from build123d import *

# Parameters (mm, degrees)
BOSS_EXTRUDE2_DEPTH = 32
CUT_EXTRUDE2_DEPTH  = 2
CHAMFER3_SIZE       = 2
CUT_EXTRUDE3_DEPTH  = 2
BOSS_EXTRUDE4_DEPTH = 2
CHAMFER4_SIZE       = 2
CUT_EXTRUDE4_DEPTH  = 2
CUT_EXTRUDE5_DEPTH  = 30


with BuildPart() as part:
    # Sketch1 → Boss-Extrude2 (new body)
    with BuildSketch(Plane(origin=(0, 0, 0), x_dir=(1, 0, 0), z_dir=(0, 1, 0))):
        Polygon((-46.372280014218745, 14.680854952562456), (-42.04215299529653, 12.180854952562488), (-43.04215299529651, 10.448804144993609), (-47.372280014218724, 12.948804144993577), (-48.37228001421871, 11.216753337424702), (-36.60670775986293, 4.423897029202528), (1.0929e-13, -2.030853223771254), (36.60670775986312, 4.423897029202558), (48.37228001421891, 11.216753337424812), (47.37228001421898, 12.948804144993561), (43.04215299529678, 10.448804144993572), (42.04215299529679, 12.180854952562449), (46.37228001421899, 14.680854952562438), (45.372280014219, 16.412905760131313), (40, 13.31121844775995), (40, 8.692416294243028), (35.91211504919529, 6.332274817479665), (0, 0), (-35.91211504919526, 6.3322748174796235), (-40.00000000000001, 8.692416294243028), (-40.00000000000001, 13.311218447759854), (-45.37228001421887, 16.41290576013115), align=None)
    extrude(amount=BOSS_EXTRUDE2_DEPTH)

    # Sketch9 → Cut-Extrude2 (cut)
    with BuildSketch(Plane(origin=(6.236073334457828, 0, 10.801195855006485), x_dir=(-0.8660254037844402, 0, 0.4999999999999974), z_dir=(-0.4999999999999974, 0, -0.8660254037844402))):
        Polygon((-44.8209624184392, 20), (-47.50000000000022, 7.944330883818674), (-47.50000000000013, 32), (-44.8209624184392, 32), align=None)
    extrude(amount=-CUT_EXTRUDE2_DEPTH, mode=Mode.SUBTRACT)

    # Chamfer3
    chamfer3_edges = [part.edges().sort_by_distance(p)[0] for p in [
        (47.872280014218944, 0, -12.082778741209186),
        (-47.87228001421872, 0, -12.08277874120914),
    ]]
    chamfer(chamfer3_edges, length=CHAMFER3_SIZE)

    # Sketch8 → Cut-Extrude3 (cut)
    with BuildSketch(Plane(origin=(-6.236073334457578, 0, 10.801195855006183), x_dir=(-0.8660254037844388, 0, -0.49999999999999983), z_dir=(0.4999999999999998, 0, -0.8660254037844387))):
        Polygon((44.82096241843918, 32), (47.50000000000006, 32), (47.50000000000006, 7.944330883819361), (44.82096241843918, 20), align=None)
    extrude(amount=-CUT_EXTRUDE3_DEPTH, mode=Mode.SUBTRACT)

    # Sketch11 → Boss-Extrude4 (add)
    with BuildSketch(Plane(origin=(0, 32, 0), x_dir=(1, 0, 0), z_dir=(0, 1, 0))):
        Polygon((-46.37228001421867, 14.680854952562523), (-45.37228001421879, 16.4129057601312), (-40.00000000000001, 13.311218447759854), (-1.3184e-13, 6.258139219421286), (40, 13.31121844775995), (45.37228001421892, 16.412905760131267), (46.372280014218916, 14.680854952562392), (45.052165410893835, 11.609285354213014), (46.05216541089376, 9.87723454664427), (36.60670775986312, 4.423897029202558), (1.0929e-13, -2.030853223771254), (-36.60670775986293, 4.423897029202528), (-46.052165410893714, 9.877234546644353), (-45.0521654108937, 11.609285354213252), align=None)
    extrude(amount=BOSS_EXTRUDE4_DEPTH)

    # Chamfer4
    chamfer4_edges = [part.edges().sort_by_distance(p)[0] for p in [
        (18.303353879931613, 34, -1.1965219027156522),
        (-18.303353879931407, 34, -1.1965219027156366),
        (41.32943658537844, 34, -7.150565787923414),
        (-41.32943658537832, 34, -7.1505657879234406),
    ]]
    chamfer(chamfer4_edges, length=CHAMFER4_SIZE)

    # Sketch12 → Cut-Extrude4 (cut)
    with BuildSketch(Plane.XZ):
        Polygon((40, -8.692416294243028), (43.04215299529678, -10.448804144993572), (47.37228001421891, -12.948804144993517), (45.37228001421892, -16.412905760131267), (40, -13.31121844775995), align=None)
        Polygon((-47.37228001421867, -12.948804144993655), (-40.00000000000001, -8.692416294243028), (-40.00000000000001, -13.311218447759854), (-45.37228001421879, -16.4129057601312), align=None)
    extrude(amount=-CUT_EXTRUDE4_DEPTH, mode=Mode.SUBTRACT)

    # Sketch13 → Cut-Extrude5 (cut)
    with BuildSketch(Plane.XZ.offset(-2)):
        Polygon((43.04215299529678, -10.448804144993572), (42.04215299529679, -12.180854952562449), (41.54215299529678, -13.046880356346884), (43.27420380286566, -14.046880356346884), (44.774203802865564, -11.448804144993552), align=None)
        Polygon((-43.04215299529651, -10.448804144993609), (-42.04215299529653, -12.180854952562488), (-41.54215299529657, -13.046880356346884), (-43.27420380286547, -14.046880356346882), (-44.77420380286537, -11.448804144993701), align=None)
    extrude(amount=-CUT_EXTRUDE5_DEPTH, mode=Mode.SUBTRACT)


solid = part.part
Read the model definition and answer for the solid it produces. Units are mm, in the model's axes. A direction names the side the tool comes from. Coordinates: 2 decimals unless noted, no trailing zeros. Loops run counter-clockwise (first coordinate to the right, second up) from the corner with the lowest first, then second, coordinate; pieces in that order, holes last.
Q1. Consider probe 1 along X at (y, z) = (16.5, -11); probe 2 along X at (y, z) = (31.5, -13.5); probe 3 along Y at (x, z) = (41.5, -13). Determine where each line is inside the solid, lowest interval first.
Q2. The part is cut by section D-D on y = 27.5. Write down the section's boundary in (x, z), and give its area (3 significant figures).
Q3. Each of these flat-tipped pins is pushed along its axis until it touches: pin 1 Ø5 at (y, z) = (19.5, -2.5) entering from -X; pin 2 Ø1 at (y, z) = (7, -7.5) entering from -X; pin 3 Ø4 at (y, z) = (15, -7) entering from -X. Where does it stop, or does it pass through?
Q4. Which of the six approach directions +Z, -Z, +X, -X, +Y, -Y give full straight-line access (tool end or side, diameter ignored) to faces 5 (the face through (46.689, 14.057, -11.416)), 6 (the face through (42.65, 17.78, -14.84)), 7 (the face through (-17.7, 15.78, -3.12)), 8 (the face through (-44, 32, -13))?
Q5. The part is cut by section A-A on y = 6. Write down the section's boundary in (x, z).
Q6. The mould has two halves that part along X. Classify faces 1 (the face through (18.56, 15.78, -1.24)), 2 (the face through (18.21, 15.78, -3.21)), 3 (the face through (-40.8, 33, -8)), 4 (the face through (42.303, 16.79, -11.73)): +X half, -X half, draft (parallel to the pull), parting line (faces both ways), or undercut.
Q7. The part is cut by section C-C on z = -3.25. Write down the section's boundary in (x, y), and give its area (3 significant figures).
Q8. The part is cut by section B-B on x = 38. Write down the section's boundary in (y, z).
Results below:
1. probe 1: x = -46.3 to -44, -42.72 to -40, 40 to 42.72, 44 to 46.3
1. probe 2: x = -44.33 to -43.59, -42.33 to -40.33, 40.33 to 42.33, 43.59 to 44.33
1. probe 3: y = 2 to 34
2. outline: (-46.37, -14.68) - (-45.37, -16.41) - (-40, -13.31) - (-40, -8.69) - (-35.91, -6.33) - (0, 0) - (35.91, -6.33) - (40, -8.69) - (40, -13.31) - (45.37, -16.41) - (46.37, -14.68) - (43.77, -13.18) - (43.27, -14.05) - (41.54, -13.05) - (43.04, -10.45) - (45.05, -11.61) - (46.05, -9.88) - (36.61, -4.42) - (0, 2.03) - (-36.61, -4.42) - (-46.05, -9.88) - (-45.05, -11.61) - (-43.04, -10.45) - (-41.54, -13.05) - (-43.27, -14.05) - (-43.77, -13.18) - close
2. area: 225 mm2
3. pin 1: stops at x = -37.6
3. pin 2: stops at x = -42.8
3. pin 3: stops at x = -44.53
4. face 5: +X, +Y
4. face 6: -Z, +Y, -Y
4. face 7: -Z, -Y
4. face 8: -Y
5. outline: (-48.37, -11.22) - (-47.37, -12.95) - (-43.04, -10.45) - (-41.54, -13.05) - (-43.27, -14.05) - (-43.77, -13.18) - (-46.37, -14.68) - (-45.37, -16.41) - (-40, -13.31) - (-40, -8.69) - (-35.91, -6.33) - (0, 0) - (35.91, -6.33) - (40, -8.69) - (40, -13.31) - (45.37, -16.41) - (46.37, -14.68) - (43.77, -13.18) - (43.27, -14.05) - (41.54, -13.05) - (43.04, -10.45) - (47.37, -12.95) - (48.37, -11.22) - (36.61, -4.42) - (0, 2.03) - (-36.61, -4.42) - close
6. face 1: +X half
6. face 2: undercut
6. face 3: -X half
6. face 4: undercut
7. outline: (-29.95, 0) - (-18.43, 0) - (-18.43, 32) - (18.43, 32) - (18.43, 0) - (29.95, 0) - (29.95, 32) - (18.43, 34) - (-18.43, 34) - (-29.95, 32) - close
7. area: 834 mm2
8. outline: (0, -7.54) - (32, -7.54) - (32, -12.96) - (34, -12.96) - (34, -7.54) - (32, -5.23) - (0, -5.23) - close
